from build123d import *

# Parameters (mm, degrees)
F2_DEPTH = 4
F4_DEPTH = 1
F5_R     = 0.99999
F7_DEPTH = 1.5


# Not quite as in the source:
# - a fillet or chamfer is up to 0.001 mm smaller than in the source, because OpenCascade refuses the exact size


with BuildPart() as f2:
    # F1 (on face) → F2 (new body)
    with BuildSketch(Plane.XY):
        with BuildLine():
            ThreePointArc((-9.4849269336, 12.5314274341), (-9.6870039278, 10.8628934269), (-10.2555653995, 9.2812554476))
            Line((-10.2555653995, 9.2812554476), (-11.9329496797, 5.8732198956))
            ThreePointArc((-11.9329496797, 5.8732198956), (0, -13.3), (11.9329496797, 5.8732198956))
            Line((11.9329496797, 5.8732198956), (10.2555653995, 9.2812554476))
            ThreePointArc((10.2555653995, 9.2812554476), (9.6870039278, 10.8628934269), (9.4849269336, 12.5314274341))
            Line((9.4849269336, 12.5314274341), (9.3996809366, 22.8774486305))
            ThreePointArc((9.3996809366, 22.8774486305), (0, 32.2), (-9.3996809366, 22.8774486305))
            Line((-9.3996809366, 22.8774486305), (-9.4849269336, 12.5314274341))
        make_face()
        with BuildLine():
            ThreePointArc((-9.8069582687, 9.0604577072), (-9.2004926988, 10.7475382184), (-8.9849439051, 12.5273078261))
            Line((-8.9849439051, 12.5273078261), (-8.899697908, 22.8733290225))
            ThreePointArc((-8.899697908, 22.8733290225), (0, 31.7), (8.899697908, 22.8733290225))
            Line((8.899697908, 22.8733290225), (8.9849439051, 12.5273078261))
            ThreePointArc((8.9849439051, 12.5273078261), (9.2004926988, 10.7475382184), (9.8069582687, 9.0604577072))
            Line((9.8069582687, 9.0604577072), (11.4843425489, 5.6524221551))
            ThreePointArc((11.4843425489, 5.6524221551), (0, -12.8), (-11.4843425489, 5.6524221551))
            Line((-11.4843425489, 5.6524221551), (-9.8069582687, 9.0604577072))
        make_face(mode=Mode.SUBTRACT)
    extrude(amount=F2_DEPTH)

    # F3 (on face) + F0 (on Top) → F4 (join)
    with BuildSketch(Plane.XY):
        with BuildLine():
            ThreePointArc((12.6780439059, 10.473563246), (12.314164564, 11.4858115527), (12.1848352877, 12.5536733173))
            Line((12.1848352877, 12.5536733173), (12.0995892907, 22.8996945138))
            ThreePointArc((12.0995892907, 22.8996945138), (0, 34.9), (-12.0995892907, 22.8996945138))
            Line((-12.0995892907, 22.8996945138), (-12.1848352877, 12.5536733173))
            ThreePointArc((-12.1848352877, 12.5536733173), (-12.314164564, 11.4858115527), (-12.6780439059, 10.473563246))
            Line((-12.6780439059, 10.473563246), (-14.3554281861, 7.0655276939))
            ThreePointArc((-14.3554281861, 7.0655276939), (0, -16), (14.3554281861, 7.0655276939))
            Line((14.3554281861, 7.0655276939), (12.6780439059, 10.473563246))
        make_face()
        with BuildLine():
            ThreePointArc((-8.899697908, 22.8733290225), (0, 31.7), (8.899697908, 22.8733290225))
            Line((8.899697908, 22.8733290225), (8.9849439051, 12.5273078261))
            ThreePointArc((8.9849439051, 12.5273078261), (9.2004926988, 10.7475382184), (9.8069582687, 9.0604577072))
            Line((9.8069582687, 9.0604577072), (11.4843425489, 5.6524221551))
            ThreePointArc((11.4843425489, 5.6524221551), (0, -12.8), (-11.4843425489, 5.6524221551))
            Line((-11.4843425489, 5.6524221551), (-9.8069582687, 9.0604577072))
            ThreePointArc((-9.8069582687, 9.0604577072), (-9.2004926988, 10.7475382184), (-8.9849439051, 12.5273078261))
            Line((-8.9849439051, 12.5273078261), (-8.899697908, 22.8733290225))
        make_face(mode=Mode.SUBTRACT)
    with BuildSketch(Plane.XY):
        with BuildLine():
            Line((-9.8069582687, 9.0604577072), (-11.4843425489, 5.6524221551))
            ThreePointArc((-11.4843425489, 5.6524221551), (0, -12.8), (11.4843425489, 5.6524221551))
            Line((11.4843425489, 5.6524221551), (9.8069582687, 9.0604577072))
            ThreePointArc((9.8069582687, 9.0604577072), (9.2004926988, 10.7475382184), (8.9849439051, 12.5273078261))
            Line((8.9849439051, 12.5273078261), (8.899697908, 22.8733290225))
            ThreePointArc((8.899697908, 22.8733290225), (0, 31.7), (-8.899697908, 22.8733290225))
            Line((-8.899697908, 22.8733290225), (-8.9849439051, 12.5273078261))
            ThreePointArc((-8.9849439051, 12.5273078261), (-9.2004926988, 10.7475382184), (-9.8069582687, 9.0604577072))
        make_face()
    extrude(amount=-F4_DEPTH)

    # F5 (radius 1 in the source; OpenCascade refuses exactly that, so slightly less here)
    f5_edges = [f2.edges().sort_by_distance(p)[0] for p in [
        (0, -16, -1),
        (-13.516736, 8.769545, -1),
        (-12.314165, 11.485812, -1),
        (-12.142212, 17.726684, -1),
        (0, 34.9, -1),
        (12.142212, 17.726684, -1),
        (12.314165, 11.485812, -1),
        (13.516736, 8.769545, -1),
    ]]
    fillet(f5_edges, radius=F5_R)

    # F6 (on face) → F7 (join)
    with BuildSketch(Plane.XY):
        with BuildLine():
            ThreePointArc((-12.1848352877, 12.5536733173), (-12.314164564, 11.4858115527), (-12.6780439059, 10.473563246))
            Line((-12.6780439059, 10.473563246), (-14.3554281861, 7.0655276939))
            ThreePointArc((-14.3554281861, 7.0655276939), (0, -16), (14.3554281861, 7.0655276939))
            Line((14.3554281861, 7.0655276939), (12.6780439059, 10.473563246))
            ThreePointArc((12.6780439059, 10.473563246), (12.314164564, 11.4858115527), (12.1848352877, 12.5536733173))
            Line((12.1848352877, 12.5536733173), (12.0995892907, 22.8996945138))
            ThreePointArc((12.0995892907, 22.8996945138), (0, 34.9), (-12.0995892907, 22.8996945138))
            ThreePointArc((-12.0995892907, 22.8996945138), (-10.0273713078, 17.7092586924), (-12.1848352877, 12.5536733173))
        make_face()
        with BuildLine():
            ThreePointArc((-10.2555653995, 9.2812554476), (-9.6870039278, 10.8628934269), (-9.4849269336, 12.5314274341))
            Line((-9.4849269336, 12.5314274341), (-9.3996809366, 22.8774486305))
            ThreePointArc((-9.3996809366, 22.8774486305), (0, 32.2), (9.3996809366, 22.8774486305))
            Line((9.3996809366, 22.8774486305), (9.4849269336, 12.5314274341))
            ThreePointArc((9.4849269336, 12.5314274341), (9.6870039278, 10.8628934269), (10.2555653995, 9.2812554476))
            Line((10.2555653995, 9.2812554476), (11.9329496797, 5.8732198956))
            ThreePointArc((11.9329496797, 5.8732198956), (0, -13.3), (-11.9329496797, 5.8732198956))
            Line((-11.9329496797, 5.8732198956), (-10.2555653995, 9.2812554476))
        make_face(mode=Mode.SUBTRACT)
    extrude(amount=F7_DEPTH)


solid = f2.part
Read the model definition and answer for the solid it produces. Units are mm, in the model's axes. A direction names the side the tool comes from. Give positions to 0.01 mm unless a question says otherwise; leave off trailing zeros. Write each loop counter-clockwise with the first axis right and the second up, starting at its lowest first coordinate (ties: lowest second). Pieces come first, ordered by that corner, then holes. Notation, with made-up numbers: (89.25, 49) - (120.25, 49) arc R14 ccw to (120.25, 57) - close; hole circle Ø7 at (-1.5, -25). An arc over 180 degrees is marked (long way). Return JSON: item names as keys, results as strings.
Q1. Consider line 1 along X through (y, z) = (0, 1.3); line 2 along X through (y, z) = (0, 1.55); line 3 along Z through (x, y) = (0.5, 23.5). Determine where each line is inside the solid, lowest interval first. Write a range as [from, to].
Reply:
{"line 1": "[-16, -12.8], [12.8, 16]", "line 2": "[-13.3, -12.8], [12.8, 13.3]", "line 3": "[-1, 0]"}
Q2. A cutting plane is placed at B-B, the plane x = 0. Determine the outline of the cut face in (y, z).
Reply:
{"outline": "(-16, 0) arc R1 ccw to (-15, -1) - (33.9, -1) arc R1 ccw to (34.9, 0) - (34.9, 1.5) - (32.2, 1.5) - (32.2, 4) - (31.7, 4) - (31.7, 0) - (-12.8, 0) - (-12.8, 4) - (-13.3, 4) - (-13.3, 1.5) - (-16, 1.5) - close"}
Q3. A cutting plane is placed at A-A, the plane z = 0.5. Determine the outline of the cut face in (x, y).
Reply:
{"outline": "(-14.36, 7.07) arc R16 ccw (long way) to (14.36, 7.07) - (12.68, 10.47) arc R4.8 cw to (12.18, 12.55) - (12.1, 22.9) arc R12.1 ccw to (-12.1, 22.9) arc R7.38 cw to (-12.18, 12.55) arc R4.8 cw to (-12.68, 10.47) - close; hole (-11.48, 5.65) arc R12.8 ccw (long way) to (11.48, 5.65) - (9.81, 9.06) arc R8 cw to (8.98, 12.53) - (8.9, 22.87) arc R8.9 ccw to (-8.9, 22.87) - (-8.98, 12.53) arc R8 cw to (-9.81, 9.06) - close"}
Q4. For a pull along Y with two mould halves and no side action, classify faces 1 (the face through (0, -16, 1)), 2 (the face through (-0.195, 31.698, 1.972)), 3 (the face through (-13.259, 8.613, -0.715)) as released by +Y, released by -Y, zero draft, split by the parting line, or undercut.
Reply:
{"face 1": "split by the parting line", "face 2": "undercut", "face 3": "released by +Y"}
Q5. Given P1, Ø16, axis at x = -8, y = -1.5, coming from the +Z side; P2, Ø1.5, axis at y = 28, z = 1, coming from the -X side; P3, Ø1, axis at y = 27.5, z = 0.5, coming from the +X side; P4, Ø1.1, axis at x = -11.5, y = 17.5, coming from the +Z side, each flat-ended and moving along its own axis, determine where each tip first touches the part or whether it passes through.
Reply:
{"P1": "z = 4", "P2": "x = -11.25", "P3": "x = 11.35", "P4": "z = 0"}
Q6. For faces 4 (the face through (11.841, 17.797, -0.715)), 5 (the face through (-9.206, 10.723, 1.972)), 6 (the face through (-11, 18, 0)), 7 (the face through (-11.083, 7.601, 2.732)), determine the directions among +Z, -Z, +X, -X, +Y, -Y from which every point of the face is accessible in a straight line to the end or side of a thin tool.
Reply:
{"face 4": "-Z, +X, +Y", "face 5": "+Z", "face 6": "+Z, -X", "face 7": "+Z, -X, +Y"}
